```python
from build123d import *

# Parameters (mm, degrees)
SKETCH1_R           = 12.573
EXTRUDE1_DEPTH      = 42.6212
CUT_EXTRUDE1_DEPTH  = 15.0876
SKETCH12_W          = 10.7188
SKETCH12_H          = 7.9375
S2D0011_W           = 3.4544
S2D0011_H           = 4.826
CUT_EXTRUDE10_DEPTH = 6.35
EXTRUDE2_DEPTH      = 3.556
CIRPATTERN2_COUNT   = 6
SKETCH18_W          = 6.35
SKETCH18_H          = 0.0762


with BuildPart() as part:
    # Sketch1 → Extrude1 (new body)
    with BuildSketch(Plane.XY):
        Circle(SKETCH1_R)
    extrude(amount=EXTRUDE1_DEPTH)

    # Sketch2 → Cut-Extrude1 (cut, symmetric)
    with BuildSketch(Plane(origin=(0, 0, 0), x_dir=(0, 0, 1), z_dir=(1, 0, 0))):
        with BuildLine():
            Line((36.7792, 12.573), (36.7792, 11.5951))
            ThreePointArc((36.7792, 11.5951), (36.927989755, 11.235889755), (37.2872, 11.0871))
            Line((37.2872, 11.0871), (42.6212, 11.0871))
            Line((42.6212, 11.0871), (42.6212, 12.573))
            Line((42.6212, 12.573), (36.7792, 12.573))
        make_face()
    cut_extrude1 = extrude(amount=CUT_EXTRUDE1_DEPTH, both=True, mode=Mode.SUBTRACT)

    # Sketch10 → Cut-Revolve1 (revolve, cut)
    with BuildSketch(Plane(origin=(0, 0, 0), x_dir=(0, 0, -1), z_dir=(1, 0, 0)), mode=Mode.PRIVATE) as cut_revolve1_sk:
        Polygon((-42.6212, 11.6713), (-37.2872, 11.6713), (-36.3855, 12.573), (-42.6212, 12.573), align=None)
    revolve(cut_revolve1_sk.sketch.rotate(Axis((0, 0, 42.424985), (0, 0, -1)), 90), axis=Axis((0, 0, 42.424985), (0, 0, -1)), mode=Mode.SUBTRACT)  # turned: the seam where the file's is

    # Sketch11 → Cut-Revolve2 (revolve, cut)
    with BuildSketch(Plane(origin=(0, 0, 0), x_dir=(0, 0, 1), z_dir=(1, 0, 0)), mode=Mode.PRIVATE) as cut_revolve2_sk:
        Polygon((0, 11.6713), (5.9944, 11.6713), (6.8961, 12.573), (0, 12.573), align=None)
    revolve(cut_revolve2_sk.sketch.rotate(Axis((0, 0, -0.344805), (0, 0, 1)), 270), axis=Axis((0, 0, -0.344805), (0, 0, 1)), mode=Mode.SUBTRACT)  # turned: the seam where the file's is

    # Sketch12 → Revolve1 (revolve)
    with BuildSketch(Plane(origin=(0, 0, 0), x_dir=(0, 0, -1), z_dir=(1, 0, 0)), mode=Mode.PRIVATE) as revolve1_sk:
        with Locations((-47.9806, 3.96875)):
            Rectangle(SKETCH12_W, SKETCH12_H)
    revolve(revolve1_sk.sketch.rotate(Axis((0, 0, 53.76799), (0, 0, -1)), 270), axis=Axis((0, 0, 53.76799), (0, 0, -1)))  # turned: the seam where the file's is

    # S2D0011 → Cut-Revolve3 (revolve, cut)
    with BuildSketch(Plane(origin=(-3.4544, 0, 53.213), x_dir=(-1, 0, 0), z_dir=(0, 1, 0))):
        with Locations((-1.7272, -2.286)):
            Rectangle(S2D0011_W, S2D0011_H)
    revolve(axis=Axis((0, 0, 27.017003875), (0, 0, 1)), mode=Mode.SUBTRACT)

    # Sketch15 → Cut-Extrude10 (cut)
    with BuildSketch(Plane.YX.offset(-53.34)):
        with BuildLine():
            Line((-3.524679028, 7.112), (3.524679028, 7.112))
            ThreePointArc((3.524679028, 7.112), (0, 7.9375), (-3.524679028, 7.112))
        make_face()
        with BuildLine():
            Line((-3.524679028, -7.112), (3.524679028, -7.112))
            ThreePointArc((3.524679028, -7.112), (0, -7.9375), (-3.524679028, -7.112))
        make_face()
    extrude(amount=CUT_EXTRUDE10_DEPTH, mode=Mode.SUBTRACT)

    # Sketch16 → Extrude2 (add)
    with BuildSketch(Plane.XY.offset(53.34)):
        Polygon((-3.666174209, 6.35), (3.666174209, 6.35), (7.332348419, 0), (3.666174209, -6.35), (-3.666174209, -6.35), (-7.332348419, 0), align=None)
    extrude(amount=EXTRUDE2_DEPTH)

    # Sketch17 → Cut-Revolve4 (revolve, cut)
    with BuildSketch(Plane(origin=(0, 0, 0), x_dir=(1, 0, 0), z_dir=(0, 1, 0)), mode=Mode.PRIVATE) as cut_revolve4_sk:
        Polygon((5.4991, -56.896), (7.332348419, -55.612345638), (7.332348419, -56.896), align=None)
    revolve(cut_revolve4_sk.sketch.rotate(Axis((0, 0, 56.833182718), (0, 0, -1)), 180), axis=Axis((0, 0, 56.833182718), (0, 0, -1)), mode=Mode.SUBTRACT)  # turned: the seam where the file's is

    # CirPattern2: Cut-Extrude1 ×6 about axis
    cirpattern2_axis = Axis((0, 0, 0), (0, 0, 1))
    for i in range(1, CIRPATTERN2_COUNT):
        add(cut_extrude1.rotate(cirpattern2_axis, i * 360 / CIRPATTERN2_COUNT), mode=Mode.SUBTRACT)

    # Sketch18 → Cut-Revolve5 (revolve, cut)
    with BuildSketch(Plane(origin=(0, 0, 0), x_dir=(0, 0, -1), z_dir=(1, 0, 0)), mode=Mode.PRIVATE) as cut_revolve5_sk:
        with Locations((-50.165, 7.8994)):
            Rectangle(SKETCH18_W, SKETCH18_H)
    revolve(cut_revolve5_sk.sketch.rotate(Axis((0, 0, 0), (0, 0, 1)), 90), axis=Axis((0, 0, 0), (0, 0, 1)), mode=Mode.SUBTRACT)  # turned: the seam where the file's is


solid = part.part
```
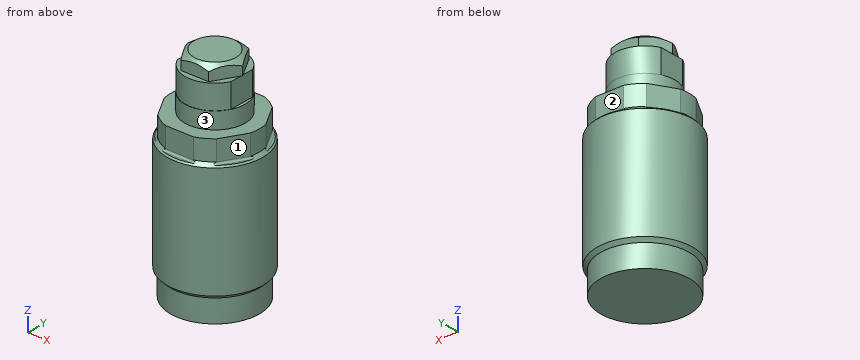
Check sheet for the modelled part. Datum: model origin and axes. Units: mm. Face numbers are marked on the shaded views. A direction names the side the tool comes from. Give positions to 0.01 mm unless a question says otherwise; leave off trailing zeros. Loops run counter-clockwise (first coordinate to the right, second up) from the corner with the lowest first, then second, coordinate; pieces in that order, holes last. Notation, with made-up numbers: (23, 39) - (82, 39) arc R19 ccw to (82, 70) - close; hole circle Ø11 at (-12.75, 58). An arc over 180 degrees is marked (long way). One line per question, with ' | ' between items. Start each with the question number.
1. Material ranges on line 1 along X through (y, z) = (0, 51.1); line 2 along Z through (x, y) = (-4, -9); line 3 along Z through (x, y) = (-3, -0.5), recorded low to high. Write a range as [from, to].
2. Set-up check for the marked faces 1, 2 and 3: record each of +Z, -Z, +X, -X, +Y, -Y from which the full face is reachable in a straight line by a thin tool's end or side.
3. Gauge pin test, flat ends, axial feed: pin 1 Ø1.5 at (x, y) = (6.5, 0) entering from +Z; pin 2 Ø3 at (x, z) = (-5.5, 13.5) entering from +Y; pin 3 Ø1.1 at (x, y) = (10.5, 5.5) entering from +Z. Record the tip position at first contact, or that the pin passes through.
4. Cross-section at A-A, the plane z = 50. Enter the section's corners in (x, y).
Check result:
1) line 1: x = [-7.11, -3.45], [3.45, 7.11] | line 2: z = [0, 42.62] | line 3: z = [0, 48.51], [53.34, 56.9]
2) face 1: +Z, +X, -Y | face 2: +Z, +X, -X, +Y | face 3: +Z
3) pin 1: stops at z = 56.72 | pin 2: stops at y = 11.92 | pin 3: stops at z = 36.88
4) outline: (-7.11, -3.35) arc R7.86 ccw to (7.11, -3.35) - (7.11, 3.35) arc R7.86 ccw to (-7.11, 3.35) - close; hole circle Ø6.91 at (0, 0)
